Geometry: final body of the model. Coordinates: model frame, mm. Give positions to 0.01 mm unless a question says otherwise; leave off trailing zeros. Write each loop counter-clockwise with the first axis right and the second up, starting at its lowest first coordinate (ties: lowest second). Pieces come first, ordered by that corner, then holes.
Q1. Cut plane A-A on y = 0. Return the cut outline in (x, z) (3 decimals), plus the area to 3 significant figures.
Q2. Line query: L1, parallel to Y at x = -0.8, z = -15.5; L2, parallel to Z at x = -0.65, y = 1.5; L3, parallel to Y at x = -0.65, z = -4.5 (3 decimals). Output: solid intervals per line, ascending.
Q3. Cut plane C-C on y = 8.5. Return the cut outline in (x, z) (1 decimal).
Q4. Cut plane D-D on y = 18.5. Return the cut outline in (x, z) (3 decimals), plus the area to 3 significant figures.
Q5. Cut plane B-B on x = -2.3. Return the cut outline in (y, z) (3 decimals).
Q6. Draft query along Y for faces 1 (the face through (-1, -36.975, 33)), 2 (the face through (-1.224, -5.544, -23.573)), 3 (the face through (-1.224, -0.813, -47.168)), 4 (the face through (-1, 1, 75.909)). Return one class per face: pulls with the +Y half, pulls with the -Y half, needs draft (parallel to the pull), parting line crosses it, or undercut.
```python
from build123d import *

# Parameters (mm, degrees)
SKETCH1_R          = 9.65
BASE_FLANGE1_DEPTH = 2.5
SCALE1_SCALE       = 1.5


# Sheet-metal steps are written as plain solids
with BuildPart() as part:
    # Sketch1 → Base-Flange1 (new body)
    with BuildSketch(Plane(origin=(0, 0, 0), x_dir=(0, 0, -1), z_dir=(1, 0, 0))):
        with BuildLine():
            Line((0, 24.65), (-57.40704, 24.65))
            Line((-57.40704, 24.65), (-57.40704, -24.65))
            Line((-57.40704, -24.65), (0, -24.65))
            ThreePointArc((0, -24.65), (24.65, 0), (0, 24.65))
        make_face()
        Circle(SKETCH1_R, mode=Mode.SUBTRACT)
    extrude(amount=-BASE_FLANGE1_DEPTH)


with BuildPart() as part_1:
    # Scale1: scaled about (-1.25, 0, 20.403540004)
    add(part.part.scale(SCALE1_SCALE).moved(Location((0.625, 0, -10.201770002))))


solid = part_1.part
```
Data:
1. outline: (-3.125, -47.177) - (0.625, -47.177) - (0.625, -24.677) - (-3.125, -24.677) - close; (-3.125, 4.273) - (0.625, 4.273) - (0.625, 75.909) - (-3.125, 75.909) - close
1. area: 353 mm2
2. L1: y = -36.59 to -13.47, 13.47 to 36.59
2. L2: z = -47.15 to -24.6, 4.2 to 75.91
2. L3: y = -36.975 to -13.305, 13.305 to 36.975
3. outline: (-3.1, -46.2) - (0.6, -46.2) - (0.6, -21.9) - (-3.1, -21.9) - close; (-3.1, 1.5) - (0.6, 1.5) - (0.6, 75.9) - (-3.1, 75.9) - close
4. outline: (-3.125, -42.216) - (0.625, -42.216) - (0.625, 75.909) - (-3.125, 75.909) - close
4. area: 443 mm2
5. outline: (-36.975, -10.202) arc R36.975 ccw to (36.975, -10.202) - (36.975, 75.909) - (-36.975, 75.909) - close; hole circle Ø28.95 at (0, -10.202)
6. face 1: pulls with the -Y half
6. face 2: undercut
6. face 3: parting line crosses it
6. face 4: needs draft
